from build123d import *

# Parameters (mm, degrees)
BOSS_EXTRUDE1_DEPTH = 10
BOSS_EXTRUDE3_DEPTH = 25
SKETCH4_R           = 5
BOSS_EXTRUDE4_DEPTH = 15
BOSS_EXTRUDE6_DEPTH = 15
MIRROR2_START       = -75
MIRROR2_DEPTH       = 50
MIRROR2_START_2     = -60
MIRROR2_2_DEPTH     = 10
MIRROR2_START_3     = -50
MIRROR2_3_OUTLINE_W = 5
MIRROR2_3_OUTLINE_H = 40
MIRROR2_3_DEPTH     = 25
MIRROR2_4_OUTLINE_R = 5
MIRROR2_4_DEPTH     = 15


# Read off the part's stored shape, not the designer's step: Mirror2
with BuildPart() as part:
    # Sketch1 → Boss-Extrude1 (new body)
    with BuildSketch(Plane(origin=(0, 0, 0), x_dir=(0, 0, -1), z_dir=(1, 0, 0))):
        with BuildLine():
            Line((-5, 61.125310432), (5, 61.125310432))
            ThreePointArc((5, 61.125310432), (15.606601718, 56.73191215), (20, 46.125310432))
            Line((20, 46.125310432), (20, 1.125310432))
            Line((20, 1.125310432), (140, -8.874689568))
            Line((140, -8.874689568), (140, -18.874689568))
            Line((140, -18.874689568), (-70.549785689, -18.874689568))
            Line((-70.549785689, -18.874689568), (-70.549785689, -8.874689568))
            Line((-70.549785689, -8.874689568), (-20, 1.125310432))
            Line((-20, 1.125310432), (-20, 46.125310432))
            ThreePointArc((-20, 46.125310432), (-15.606601718, 56.73191215), (-5, 61.125310432))
        make_face()
    extrude(amount=BOSS_EXTRUDE1_DEPTH)

    # Sketch3 → Boss-Extrude3 (add)
    with BuildSketch(Plane.ZY):
        Polygon((20, 1.125310432), (70.549785689, -8.874689568), (70.549785689, -18.874689568), (-140, -18.874689568), (-140, -8.874689568), (-20, 1.125310432), (-20, 6.125310432), (20, 6.125310432), align=None)
    extrude(amount=BOSS_EXTRUDE3_DEPTH)

    # Sketch4 → Boss-Extrude4 (add)
    with BuildSketch(Plane(origin=(10, 0, 0), x_dir=(0, 0, -1), z_dir=(1, 0, 0))):
        with Locations(Location((0, 41.125310432, 0), (0, 0, 180))):
            Circle(SKETCH4_R)
    extrude(amount=BOSS_EXTRUDE4_DEPTH)

    # Sketch7 → Boss-Extrude6 (add)
    with BuildSketch(Plane(origin=(10, 0, 0), x_dir=(0, 0, -1), z_dir=(1, 0, 0))):
        Polygon((-70.549785689, -8.874689568), (-20, 1.125310432), (20, 1.125310432), (140, -8.874689568), (140, -18.874689568), (-70.549785689, -18.874689568), align=None)
    extrude(amount=BOSS_EXTRUDE6_DEPTH)

    # Mirror2 outline → Mirror2 (add)
    with BuildSketch(Plane.YZ.offset(MIRROR2_START)):
        Polygon((-8.874689568, 70.549785689), (-18.874689568, 70.549785689), (-18.874689568, -140), (-8.874689568, -140), (1.125310432, -20), (1.125310432, 20), align=None)
    extrude(amount=MIRROR2_DEPTH)

    # Mirror2 2 outline → Mirror2 2 (add)
    with BuildSketch(Plane.YZ.offset(MIRROR2_START_2)):
        with BuildLine():
            Line((1.125310432, 20), (1.125310432, -20))
            Line((1.125310432, -20), (46.125310432, -20))
            ThreePointArc((46.125310432, -20), (56.73191215, -15.606601718), (61.125310432, -5))
            Line((61.125310432, -5), (61.125310432, 5))
            ThreePointArc((61.125310432, 5), (56.73191215, 15.606601718), (46.125310432, 20))
            Line((46.125310432, 20), (1.125310432, 20))
        make_face()
    extrude(amount=MIRROR2_2_DEPTH)

    # Mirror2 3 outline → Mirror2 3 (add)
    with BuildSketch(Plane.YZ.offset(MIRROR2_START_3)):
        with Locations((3.625310432, 0)):
            Rectangle(MIRROR2_3_OUTLINE_W, MIRROR2_3_OUTLINE_H)
    extrude(amount=MIRROR2_3_DEPTH)

    # Mirror2 4 outline → Mirror2 4 (add)
    with BuildSketch(Plane.YZ.offset(MIRROR2_START)):
        with Locations((41.125310432, 0)):
            Circle(MIRROR2_4_OUTLINE_R)
    extrude(amount=MIRROR2_4_DEPTH)


solid = part.part
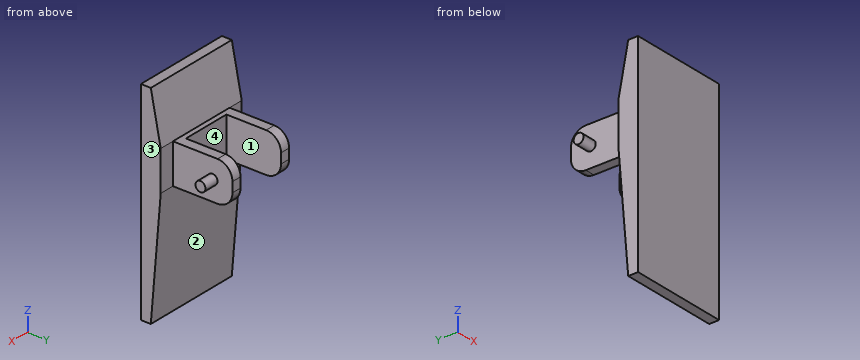
Design review of the part built by this model. Coordinates are the model's own, in mm. Face numbers are marked on the shaded views. Coordinates: 2 decimals unless noted, no trailing zeros. Order: outer loops, then holes, each group sorted by start corner. A loop starts at its lowest first (then second) coordinate and runs counter-clockwise, first axis right, second up.
Item 1: For line 1 (X direction, y = 19.5, z = -12); line 2 (Y direction, x = -8, z = 3); line 3 (Z direction, x = 8, y = 31), list the stretches that pass through material, from the lowest coordinate up.
Item 2: Take a section at A-A, the plane x = -65.5. Write out the cut boundary in (y, z).
Item 3: Take a section at C-C, the plane z = 0. Write out the cut boundary in (x, y).
Item 4: Take a section at D-D, the plane x = -39. Write out the cut boundary in (y, z).
Item 5: For pin 1 Ø8 at (y, z) = (24, -2) entering from -X; pin 2 Ø22.5 at (x, y) = (-18, 32) entering from +Z; pin 3 Ø7.5 at (x, z) = (-66, -8) entering from +Y; pin 4 Ø4.5 at (x, z) = (16, -2) entering from +Y, all flat-tipped, find the tip position at first contact; note any pin that passes through.
Item 6: The part is to be moulded in two halves that separate along X. For the marked faces 1, 2, 3 and 4, say which applies: pulls with the +X half, pulls with the -X half, needs draft (parallel to the pull), parting line crosses it, or undercut.
Item 7: Take a section at B-B, the plane y = 27. Write out the cut boundary in (x, z).
The answers:
1. line 1: x = -60 to -50, 0 to 10
1. line 2: y = -18.87 to 6.13
1. line 3: z = -20 to 20
2. outline: (-18.87, -140) - (-8.87, -140) - (1.13, -20) - (1.13, 20) - (-8.87, 70.55) - (-18.87, 70.55) - close; circle Ø10 at (41.13, 0)
3. outline: (-75, -18.87) - (25, -18.87) - (25, 1.13) - (10, 1.13) - (10, 36.13) - (25, 36.13) - (25, 46.13) - (10, 46.13) - (10, 61.13) - (0, 61.13) - (0, 6.13) - (-50, 6.13) - (-50, 61.13) - (-60, 61.13) - (-60, 46.13) - (-75, 46.13) - (-75, 36.13) - (-60, 36.13) - (-60, 1.13) - (-75, 1.13) - close
4. outline: (-18.87, -140) - (-8.87, -140) - (1.13, -20) - (6.13, -20) - (6.13, 20) - (1.13, 20) - (-8.87, 70.55) - (-18.87, 70.55) - close
5. pin 1: stops at x = -60
5. pin 2: passes through
5. pin 3: stops at y = 43.76
5. pin 4: stops at y = 46.13
6. face 1: undercut
6. face 2: needs draft
6. face 3: pulls with the +X half
6. face 4: undercut
7. outline: (-60, -20) - (-50, -20) - (-50, 20) - (-60, 20) - close; (0, -20) - (10, -20) - (10, 20) - (0, 20) - close
